Check sheet for the drawn part. Datum: minimum x, y, z corner. Units: mm. A direction names the side the tool comes from. Coordinates: 2 decimals unless noted, no trailing zeros. Order: outer loops, then holes, each group sorted by start corner. A loop starts at its lowest first (then second) coordinate and runs counter-clockwise, first axis right, second up.
1. Set-up check for the marked faces 5 and 6: record each of +Z, -Z, +X, -X, +Y, -Y from which the full face is reachable in a straight line by a thin tool's end or side.
2. Thickness scan on line 1 (Z direction, x = 19, y = 31); line 2 (Y direction, x = 63.5, z = 71); line 3 (X direction, y = 17.5, z = 35.5) (1 decimal). Record the ranges inside material, lowest first.
3. Draft check along X on the marked faces 1, 2, 3 and 4. Enter one of: released by +X, released by -X, zero draft, split by the parting line, or undercut.
4. Cross-section at B-B (y = 24.5). Enter the section's corners in (x, z) (1 decimal).
5. Cross-section at A-A (x = 60). Enter the section's corners in (y, z), then the cut area to 3 significant figures.
6. Gauge pin test, flat ends, axial feed: pin 1 Ø2 at (x, z) = (39, 46.5) entering from -Y; pin 2 Ø1.5 at (x, y) = (40.5, 8.5) entering from +Z. Record the tip position at first contact, or that the pin passes through.
7. Cross-section at C-C (z = 25). Enter the section's corners in (x, y) (1 decimal).
8. Cross-section at D-D (z = 59). Enter the section's corners in (x, y) (1 decimal).
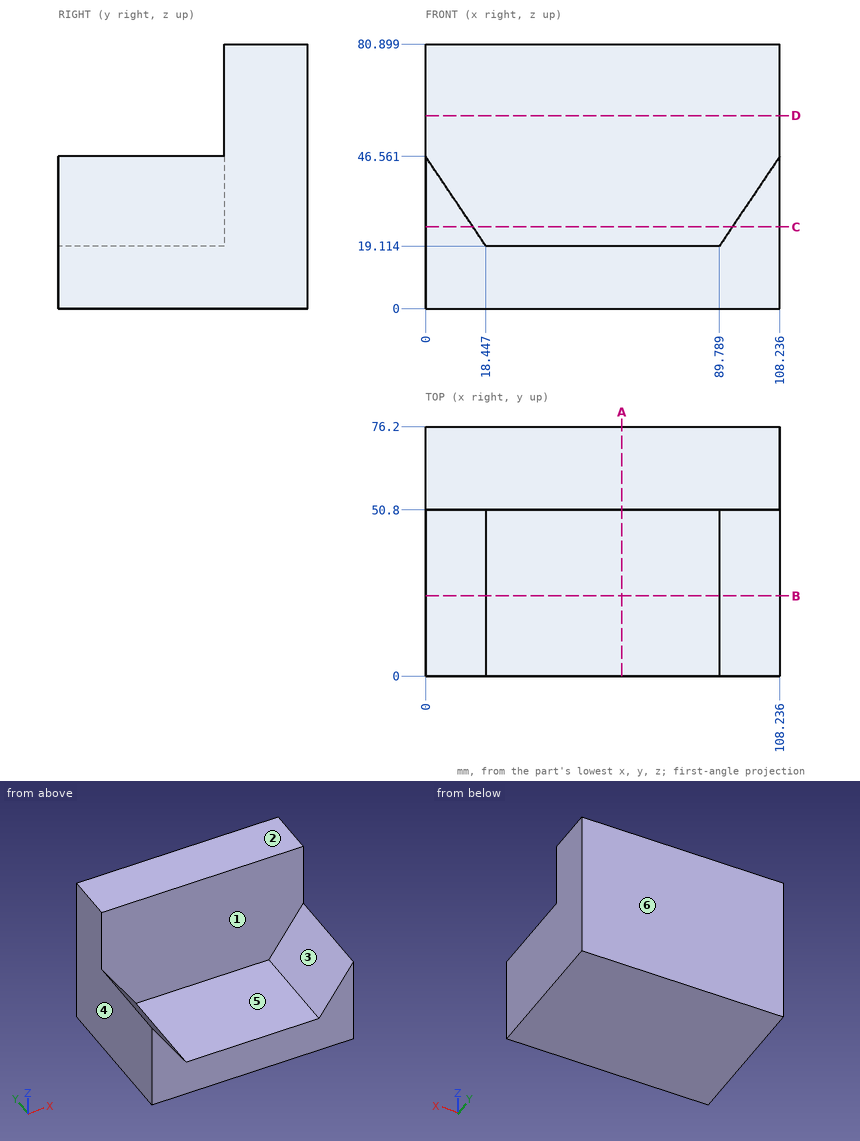
Data:
1. face 5: +Z, -Y
1. face 6: +Z, -Z, +X, -X, +Y
2. line 1: z = 0 to 19.11
2. line 2: y = 50.8 to 76.2
2. line 3: x = 0 to 7.4, 100.8 to 108.2
3. face 1: undercut
3. face 2: zero draft
3. face 3: undercut
3. face 4: released by -X
4. outline: (0, 0) - (108.2, 0) - (108.2, 46.6) - (89.8, 19.1) - (18.4, 19.1) - (0, 46.6) - close
5. outline: (0, 0) - (76.2, 0) - (76.2, 80.9) - (50.8, 80.9) - (50.8, 19.11) - (0, 19.11) - close
5. area: 3,030 mm2
6. pin 1: stops at y = 50.8
6. pin 2: stops at z = 19.11
7. outline: (0, 0) - (14.5, 0) - (14.5, 50.8) - (93.7, 50.8) - (93.7, 0) - (108.2, 0) - (108.2, 76.2) - (0, 76.2) - close
8. outline: (0, 50.8) - (108.2, 50.8) - (108.2, 76.2) - (0, 76.2) - close
